Check sheet for the modelled part. Datum: model origin and axes. Units: mm. A direction names the side the tool comes from. Round coordinates to 2 decimals unless told otherwise and drop trailing zeros. Write each loop counter-clockwise with the first axis right and the second up, starting at its lowest first coordinate (ties: lowest second). Pieces come first, ordered by that corner, then holes. Notation, with made-up numbers: M 37,27.5 L 42,27.5 A29 cw 42,47.5 Z; hole C -39,70.25 d4. An arc over 180 degrees is marked long. One line per item, written item: value.
from build123d import *

# Parameters (mm, degrees)
SKETCH1_W           = 145
SKETCH1_H           = 90
BOSS_EXTRUDE1_DEPTH = 5
SKETCH3_W           = 120
SKETCH3_H           = 34.25
CUT_EXTRUDE1_DEPTH  = 5
SKETCH4_W           = 5
SKETCH4_H           = 40.8
SKETCH4_H_2         = 23.1
CUT_EXTRUDE2_DEPTH  = 5
SKETCH7_W           = 50.2
SKETCH7_H           = 5
CUT_EXTRUDE3_DEPTH  = 5
SKETCH9_R           = 1.5
CUT_EXTRUDE4_DEPTH  = 10


with BuildPart() as part:
    # Sketch1 → Boss-Extrude1 (new body)
    with BuildSketch(Plane(origin=(0, 0, 0), x_dir=(1, 0, 0), z_dir=(0, 1, 0))):
        Rectangle(SKETCH1_W, SKETCH1_H)
    extrude(amount=BOSS_EXTRUDE1_DEPTH)

    # Sketch3 → Cut-Extrude1 (cut)
    with BuildSketch(Plane(origin=(0, 5, 0), x_dir=(1, 0, 0), z_dir=(0, 1, 0))):
        with Locations((0, -7.365)):
            Rectangle(SKETCH3_W, SKETCH3_H)
    extrude(amount=-CUT_EXTRUDE1_DEPTH, mode=Mode.SUBTRACT)

    # Sketch4 → Cut-Extrude2 (cut)
    with BuildSketch(Plane(origin=(0, 5, 0), x_dir=(1, 0, 0), z_dir=(0, 1, 0))):
        with Locations((-70, 24.6)):
            Rectangle(SKETCH4_W, SKETCH4_H)
        with Locations((-70, -33.45)):
            Rectangle(SKETCH4_W, SKETCH4_H_2)
        with Locations((70, -33.45)):
            Rectangle(SKETCH4_W, SKETCH4_H_2)
        with Locations((70, 24.6)):
            Rectangle(SKETCH4_W, SKETCH4_H)
    extrude(amount=-CUT_EXTRUDE2_DEPTH, mode=Mode.SUBTRACT)

    # Sketch7 → Cut-Extrude3 (cut)
    with BuildSketch(Plane(origin=(0, 5, 0), x_dir=(1, 0, 0), z_dir=(0, 1, 0))):
        with Locations((0, -42.5)):
            Rectangle(SKETCH7_W, SKETCH7_H)
    extrude(amount=-CUT_EXTRUDE3_DEPTH, mode=Mode.SUBTRACT)

    # Sketch9 → Cut-Extrude4 (cut)
    with BuildSketch(Plane(origin=(0, 5, 0), x_dir=(1, 0, 0), z_dir=(0, 1, 0))):
        with Locations(Location((-58, 33.5, 0), (0, 0, 270))):
            Circle(SKETCH9_R)
        with Locations(Location((58, 33.5, 0), (0, 0, 270))):
            Circle(SKETCH9_R)
        with Locations(Location((58, -33.5, 0), (0, 0, 270))):
            Circle(SKETCH9_R)
        with Locations(Location((-58, -33.5, 0), (0, 0, 270))):
            Circle(SKETCH9_R)
    extrude(amount=-CUT_EXTRUDE4_DEPTH, mode=Mode.SUBTRACT)


solid = part.part
Q1. Draft check along X on faces 1 (the flat face through (-1, 0, -11)), 2 (the flat face through (-72.5, 2, 9)), 3 (the flat face through (-1, 3, 24.49)). Enter one of: pulls with the +X half, pulls with the -X half, needs draft (parallel to the pull), parting line crosses it, or undercut.
Completed:
face 1: needs draft
face 2: pulls with the -X half
face 3: undercut
Q2. Sectioned sample at B-B on x = 17.5. Enter the section's corners in (y, z).
Completed:
outline: M 0,-45 L 5,-45 L 5,-9.76 L 0,-9.76 Z; M 0,24.49 L 5,24.49 L 5,40 L 0,40 Z
Q3. Sectioned sample at D-D on y = 2.8. Enter the section's corners in (x, z), and give its area (3 significant figures).
Completed:
outline: M -72.5,-4.2 L -67.5,-4.2 L -67.5,-45 L 67.5,-45 L 67.5,-4.2 L 72.5,-4.2 L 72.5,21.9 L 67.5,21.9 L 67.5,45 L 25.1,45 L 25.1,40 L -25.1,40 L -25.1,45 L -67.5,45 L -67.5,21.9 L -72.5,21.9 Z; hole M -60,-9.76 L 60,-9.76 L 60,24.49 L -60,24.49 Z; hole C -58,-33.5 d3; hole C -58,33.5 d3; hole C 58,-33.5 d3; hole C 58,33.5 d3
area: 8,020 mm^2
Q4. Scan lines: line 1 (X direction, y = 3.65, z = -33.5); line 2 (Z direction, x = 55, y = 0.5); line 3 (Z direction, x = -5, y = 1.45). Record each from-to range of solid material in increasing order. Write a range as [from, to].
Completed:
line 1: [-67.5, -59.5], [-56.5, 56.5], [59.5, 67.5]
line 2: [-45, -9.76], [24.49, 45]
line 3: [-45, -9.76], [24.49, 40]
Q5. Access from +Z, -Z, +X, -X, +Y, -Y to the whole of each face (thin tool, end or side, straight path). Record for faces 4 (the flat face through (70, 3, -4.2)), 5 (the flat face through (0, 3, 40)), 6 (the flat face through (-67.5, 3, 34)), 7 (the flat face through (70, 3, 21.9)), 8 (the flat face through (60, 3, 8)).
Completed:
face 4: -Z, +X, +Y, -Y
face 5: +Z, +Y, -Y
face 6: +Z, -X, +Y, -Y
face 7: +Z, +X, +Y, -Y
face 8: +Y, -Y
Q6. Depth check by flat-ended pin: P1, Ø4, axis at x = 58, z = -33.5, coming from the +Y side; P2, Ø2.5, axis at x = -69, y = 2, coming from the +Z side; P3, Ø1.8, axis at x = -58, z = 33.5, coming from the +Y side; P4, Ø1.5, axis at y = 4.5, z = 33, coming from the -X side. Enter the tip coordinate at first touch or a pass-through.
Completed:
P1: y = 5
P2: z = 21.9
P3: through
P4: x = -67.5
Q7. Sectioned sample at A-A on z = 3. Enter the section's corners in (x, y).
Completed:
outline: M -72.5,0 L -60,0 L -60,5 L -72.5,5 Z; M 60,0 L 72.5,0 L 72.5,5 L 60,5 Z
Q8. Sectioned sample at C-C on z = -33.5. Enter the section's corners in (x, y).
Completed:
outline: M -67.5,0 L -59.5,0 L -59.5,5 L -67.5,5 Z; M -56.5,0 L 56.5,0 L 56.5,5 L -56.5,5 Z; M 59.5,0 L 67.5,0 L 67.5,5 L 59.5,5 Z
